from build123d import *

# Parameters (mm, degrees)
SKETCH1_W           = 85
SKETCH1_H           = 56
SKETCH1_R           = 1.5
BOSS_EXTRUDE1_DEPTH = 1.5
SKETCH2_W           = 25
SKETCH2_H           = 15
SKETCH2_W_2         = 20
SKETCH2_H_2         = 12
BOSS_EXTRUDE2_DEPTH = 8


with BuildPart() as part:
    # Sketch1 → Boss-Extrude1 (new body)
    with BuildSketch(Plane.XY):
        Rectangle(SKETCH1_W, SKETCH1_H)
        with Locations((-39, 24.5)):
            Circle(SKETCH1_R, mode=Mode.SUBTRACT)
        with Locations((19, 24.5)):
            Circle(SKETCH1_R, mode=Mode.SUBTRACT)
        with Locations((19, -24.5)):
            Circle(SKETCH1_R, mode=Mode.SUBTRACT)
        with Locations((-39, -24.5)):
            Circle(SKETCH1_R, mode=Mode.SUBTRACT)
    extrude(amount=BOSS_EXTRUDE1_DEPTH)

    # Sketch2 → Boss-Extrude2 (add)
    with BuildSketch(Plane.XY.offset(1.5)):
        with Locations((36, -17.8)):
            Rectangle(SKETCH2_W, SKETCH2_H)
        with Locations((38.5, 1.1)):
            Rectangle(SKETCH2_W_2, SKETCH2_H_2)
        with Locations((38.5, 19)):
            Rectangle(SKETCH2_W_2, SKETCH2_H_2)
    extrude(amount=BOSS_EXTRUDE2_DEPTH)


solid = part.part
Verification items for the finished model (mm, model axes). A direction names the side the tool comes from. Give positions to 0.01 mm unless a question says otherwise; leave off trailing zeros. Order: outer loops, then holes, each group sorted by start corner. A loop starts at its lowest first (then second) coordinate and runs counter-clockwise, first axis right, second up. Notation, with made-up numbers: M -4,-19 L 41,-19 A20 ccw 41,-14 Z; hole C 33,61 d3. An arc over 180 degrees is marked long. Answer as a JSON object with one key per item and string values. Group by question number.
1) Cross-section at D-D (x = 35). Enter the section's corners in (y, z).
2) Cross-section at B-B (x = -39). Enter the section's corners in (y, z).
3) Cross-section at C-C (y = -12.5). Enter the section's corners in (x, z).
4) Access from +Z, -Z, +X, -X, +Y, -Y to the whole of each face (thin tool, end or side, straight path). Record for faces 1 (the face through (23.5, -18, 5)), 2 (the face through (45, -18, 1.5)), 3 (the face through (-40.11, -23.49, 0.74)), 4 (the face through (28.5, 19, 5)), 5 (the face through (38, -4.9, 5)).
5) Cross-section at A-A (z = 8.5). Enter the section's corners in (x, y), then the cut area to 3 significant figures.
6) Scan lines: line 1 along Y through (x, z) = (35, 3); line 2 along Y through (x, z) = (19, 1); line 3 along Z through (x, y) = (20, -0.5). Record each from-to range of solid material in increasing order. Write a range as [from, to].
7) Depth check by flat-ended pin: pin 1 Ø3 at (x, y) = (46.5, -1.5) entering from -Z; pin 2 Ø4 at (y, z) = (-16, 4) entering from -X; pin 3 Ø4 at (y, z) = (16, 6.5) entering from -X. Enter the tip coordinate at first touch or a pass-through.
8) Mould release check, pull along Y, two halves, no side actions. Record for faces 6 (the face through (38, 7.1, 5)), 7 (the face through (36, -25.3, 5)), 8 (the face through (38, 1, 9.5)): released by +Y, released by -Y, zero draft, split by the parting line, or undercut.
Result sheet:
{
 "1": {"outline": "M -28,0 L 28,0 L 28,1.5 L 25,1.5 L 25,9.5 L 13,9.5 L 13,1.5 L 7.1,1.5 L 7.1,9.5 L -4.9,9.5 L -4.9,1.5 L -10.3,1.5 L -10.3,9.5 L -25.3,9.5 L -25.3,1.5 L -28,1.5 Z"},
 "2": {"outline": "M -28,0 L -26,0 L -26,1.5 L -28,1.5 Z; M -23,0 L 23,0 L 23,1.5 L -23,1.5 Z; M 26,0 L 28,0 L 28,1.5 L 26,1.5 Z"},
 "3": {"outline": "M -42.5,0 L 42.5,0 L 42.5,1.5 L 48.5,1.5 L 48.5,9.5 L 23.5,9.5 L 23.5,1.5 L -42.5,1.5 Z"},
 "4": {"face 1": "+Z, -X, +Y, -Y", "face 2": "-Z, +X, +Y, -Y", "face 3": "+Z, -Z", "face 4": "+Z, -X, +Y", "face 5": "+Z, +X, -X"},
 "5": {"outline": "M 23.5,-25.3 L 48.5,-25.3 L 48.5,-10.3 L 23.5,-10.3 Z; M 28.5,-4.9 L 48.5,-4.9 L 48.5,7.1 L 28.5,7.1 Z; M 28.5,13 L 48.5,13 L 48.5,25 L 28.5,25 Z", "area": "855 mm2"},
 "6": {"line 1": "y = [-25.3, -10.3], [-4.9, 7.1], [13, 25]", "line 2": "y = [-28, -26], [-23, 23], [26, 28]", "line 3": "z = [0, 1.5]"},
 "7": {"pin 1": "stops at z = 1.5", "pin 2": "stops at x = 23.5", "pin 3": "stops at x = 28.5"},
 "8": {"face 6": "undercut", "face 7": "released by -Y", "face 8": "zero draft"}
}
